Model file for the job. Use its own axes, mm. A direction names the side the tool comes from. Give positions to 0.01 mm unless a question says otherwise; leave off trailing zeros. Order: outer loops, then holes, each group sorted by start corner. A loop starts at its lowest first (then second) coordinate and runs counter-clockwise, first axis right, second up. Notation, with made-up numbers: (-23.5, -30) - (-15.5, -30) arc R18 ccw to (-15.5, -5) - close; hole circle Ø8 at (68, 38.25). An arc over 180 degrees is marked (long way). Return JSON: item names as keys, results as strings. Group by question number.
from build123d import *

# Parameters (mm, degrees)
BOSS_EXTRUDE1_DEPTH      = 36.825
BOSS_EXTRUDE1_DEPTH_BACK = 3.175
BOSS_EXTRUDE2_DEPTH      = 33.65


with BuildPart() as part:
    # Sketch1 → Boss-Extrude1 (new, two sides: drawn at the far end of the back side and taken through both)
    with BuildSketch(Plane.XY.offset(-BOSS_EXTRUDE1_DEPTH_BACK)):
        with BuildLine():
            Line((6.103170523, 84.664670477), (7.148138473, 92.601990083))
            ThreePointArc((7.148138473, 92.601990083), (6.704979898, 94.139454624), (5.276321506, 94.859955796))
            ThreePointArc((5.276321506, 94.859955796), (0, 95.006582836), (-5.276321506, 94.859955796))
            ThreePointArc((-5.276321506, 94.859955796), (-6.704979898, 94.139454624), (-7.148138473, 92.601990083))
            Line((-7.148138473, 92.601990083), (-6.103170523, 84.664670477))
            ThreePointArc((-6.103170523, 84.664670477), (-5.402140732, 83.39052414), (-4.023362223, 82.928072545))
            ThreePointArc((-4.023362223, 82.928072545), (0, 83.025614479), (4.023362223, 82.928072545))
            ThreePointArc((4.023362223, 82.928072545), (5.402140732, 83.39052414), (6.103170523, 84.664670477))
        make_face()
    extrude(amount=BOSS_EXTRUDE1_DEPTH + BOSS_EXTRUDE1_DEPTH_BACK)

    # Sketch2 → Boss-Extrude2 (add)
    with BuildSketch(Plane.XY):
        with BuildLine():
            Line((7.094615384, 84.534144285), (8.139583334, 92.47146389))
            ThreePointArc((8.139583334, 92.47146389), (7.474845471, 94.777660702), (5.331857885, 95.85841246))
            ThreePointArc((5.331857885, 95.85841246), (0, 96.006582836), (-5.331857885, 95.85841246))
            ThreePointArc((-5.331857885, 95.85841246), (-7.474845471, 94.777660702), (-8.139583334, 92.47146389))
            Line((-8.139583334, 92.47146389), (-7.094615384, 84.534144285))
            ThreePointArc((-7.094615384, 84.534144285), (-6.043070698, 82.622924779), (-3.974902934, 81.929247386))
            ThreePointArc((-3.974902934, 81.929247386), (0, 82.025614479), (3.974902934, 81.929247386))
            ThreePointArc((3.974902934, 81.929247386), (6.043070698, 82.622924779), (7.094615384, 84.534144285))
        make_face()
    extrude(amount=BOSS_EXTRUDE2_DEPTH)


solid = part.part
(1) 3-axis set-ups, long thin cutter, end or side, ignore diameter. For faces 4 (the face through (-0.056, 82.026, 16.589)), 5 (the face through (1.2, 95.3, 33.65)), 6 (the face through (6.62, 88.58, -1.61)), 7 (the face through (-6.633, 88.689, -1.61)), 8 (the face through (6.62, 88.58, 35.22)): which of +Z, -Z, +X, -X, +Y, -Y reach the whole face in a straight line?
(2) Slice it at A-A (x = -4.5). Give the cut face in (y, z) (3 decimals), and give its area (3 significant figures).
(3) Drill centre lines: L1, parallel to Y at x = -0.75, z = 21; L2, parallel to Z at x = 6.5, y = 83.5; L3, parallel to X at y = 85, z = 5. Where is each one in solid material? Low to high.
(4) Pull direction Y, two halves, no side cores. Call faces 1 (the face through (1.2, 95.3, 0)), 2 (the face through (0.074, 95.007, 35.215)), 3 (the face through (-0.056, 83.026, -1.61)): released by +Y, released by -Y, zero draft, split by the parting line, or undercut.
(5) Drop flat-ended pins along their axis: pin 1 Ø1.5 at (y, z) = (90, 15.5) entering from +X; pin 2 Ø4 at (y, z) = (85.5, 16) entering from +X; pin 3 Ø1 at (y, z) = (85.5, 24) entering from -X. Give the stop position or say it passes through.
(6) Slice it at C-C (y = 91). Give the cut face in (x, z) (3 decimals).
(7) Slice it at B-B (z = 11). Give the cut face in (x, y).
Result set:
{
 "1": {"face 4": "+Z, -Z, -Y", "face 5": "+Z", "face 6": "-Z, +X, -Y", "face 7": "-Z, -X, -Y", "face 8": "+Z, +X, -Y"},
 "2": {"outline": "(81.95, 0) - (82.962, 0) - (82.962, -3.175) - (94.9, -3.175) - (94.9, 0) - (95.901, 0) - (95.901, 33.65) - (94.9, 33.65) - (94.9, 36.825) - (82.962, 36.825) - (82.962, 33.65) - (81.95, 33.65) - close", "area": "545 mm²"},
 "3": {"L1": "y = 82.02 to 96", "L2": "z = 0 to 33.65", "L3": "x = -7.16 to 7.16"},
 "4": {"face 1": "zero draft", "face 2": "released by +Y", "face 3": "released by -Y"},
 "5": {"pin 1": "stops at x = 7.91", "pin 2": "stops at x = 7.49", "pin 3": "stops at x = -7.29"},
 "6": {"outline": "(-7.946, 0) - (-6.937, 0) - (-6.937, -3.175) - (6.937, -3.175) - (6.937, 0) - (7.946, 0) - (7.946, 33.65) - (6.937, 33.65) - (6.937, 36.825) - (-6.937, 36.825) - (-6.937, 33.65) - (-7.946, 33.65) - close"},
 "7": {"outline": "(-8.14, 92.47) - (-7.09, 84.53) arc R3 ccw to (-3.97, 81.93) arc R82.03 cw to (3.97, 81.93) arc R3 ccw to (7.09, 84.53) - (8.14, 92.47) arc R3 ccw to (5.33, 95.86) arc R96.01 ccw to (-5.33, 95.86) arc R3 ccw to start"}
}
